Could you check a few things on this model? Use its own coordinates, in mm. Face numbers are marked on the shaded views. Coordinates: 2 decimals unless noted, no trailing zeros. Write each loop counter-clockwise with the first axis right and the second up, starting at its lowest first coordinate (ties: lowest second). Pieces come first, ordered by that corner, then holes.
Item 1: If I drill on probe 1 along Y at (x, z) = (0, 17.25); probe 2 along Y at (x, z) = (0, 20); probe 3 along Y at (x, z) = (-12.25, 18.2), over which ranges is the centre line in solid material (lowest first)?
Item 2: I want a section at A-A on y = 82.8. Please give me the cut outline in (x, z), then the cut area to 3 significant figures.
Item 3: I want a section at B-B on y = -0.2. Please give me the cut outline in (x, z).
Item 4: Thinking about a two-plate mould opening in X: for the marked faces 1, 2, 3 and 4, which applies, +X half, -X half, draft (parallel to the pull), parting line (faces both ways), or undercut?
Item 5: For P1, Ø1.5, axis at y = 64.5, z = 18, coming from the -X side; P2, Ø2.5, axis at x = 0, z = 18.2, coming from the +Y side, each with a flat end and sliding along its axis, tell me the tip position at first contact or that it passes through.
Item 6: I want a section at D-D on z = 18.2. State how many separate pieces and enclosed holes the cut face has, then the cut area to 3 significant figures.
Item 7: I want a section at C-C on x = 0. Please give me the cut outline in (y, z), then the cut area to 3 significant figures.
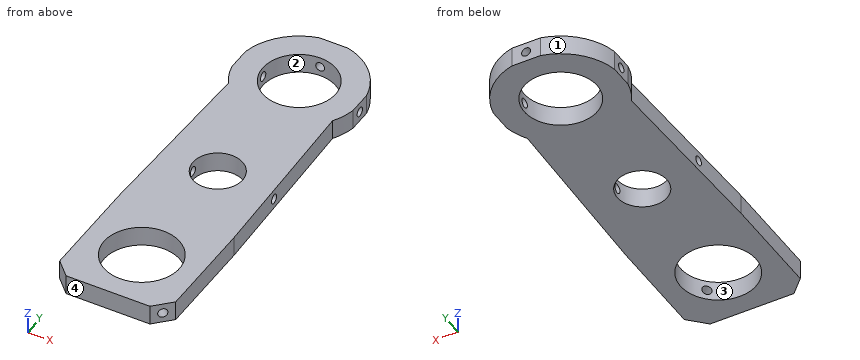
from build123d import *

# Parameters (mm, degrees)
SKETCH002_R          = 7.5
SKETCH002_R_2        = 11.4
SKETCH002_R_3        = 11
PAD002_DEPTH         = 6
SKETCH003_R          = 1.4
POCKET_DEPTH         = 20
SKETCH004_R          = 1.4
POCKET001_DEPTH      = 36.866111375
SKETCH005_R          = 1.4
POCKET002_DEPTH      = 36.6206712513
SKETCH006_R          = 1.35
POCKET003_DEPTH      = 10
BODY_PLACEMENT_ANGLE = 180


with BuildPart() as part:
    # Sketch002 → Pad002 (new body)
    with BuildSketch(Plane.XY):
        with BuildLine():
            Line((17.4185858621, -21.7716146623), (15.72, 32.8960215672))
            ThreePointArc((15.72, 32.8960215672), (17.3549083149, 36.0552761319), (18.3596204304, 39.4676606599))
            Line((18.3596204304, 39.4676606599), (18.3596204304, 46.5323393401))
            ThreePointArc((18.3596204304, 46.5323393401), (13.5034413002, 55.9064608862), (4.3329172916, 61.1369598984))
            Line((-4.3329172916, 61.1369598984), (4.3329172916, 61.1369598984))
            ThreePointArc((-4.3329172916, 61.1369598984), (-13.4407809455, 55.8794757058), (-18.2600508209, 46.5323393401))
            Line((-18.2600508209, 39.4676606599), (-18.2600508209, 46.5323393401))
            ThreePointArc((-18.2600508209, 39.4676606599), (-17.2898053647, 36.137342842), (-15.72, 33.0441076213))
            Line((-17.4185858621, -21.7716146623), (-15.72, 33.0441076213))
            Line((-17.4185858621, -52.4548343373), (-17.4185858621, -21.7716146623))
            Line((-17.4185858621, -52.4548343373), (-12.4548343373, -57.4185858621))
            Line((-12.4548343373, -57.4185858621), (12.8963534851, -57.4185858621))
            Line((17.4185858621, -52.8963534851), (12.8963534851, -57.4185858621))
            Line((17.4185858621, -52.8963534851), (17.4185858621, -21.7716146623))
        make_face()
        Circle(SKETCH002_R, mode=Mode.SUBTRACT)
        with Locations((0, -40)):
            Circle(SKETCH002_R_2, mode=Mode.SUBTRACT)
        with Locations((0.0652183529, 43)):
            Circle(SKETCH002_R_3, mode=Mode.SUBTRACT)
    extrude(amount=PAD002_DEPTH)

    # Sketch003 (on Face12 of Pad002) → Pocket (cut)
    with BuildSketch(Plane(origin=(-34.9367100997, -34.9367100997, 0), x_dir=(0.7071067812, -0.7071067812, 0), z_dir=(-0.7071067812, -0.7071067812, 0))):
        with Locations((28.2842712475, 3)):
            Circle(SKETCH003_R)
    extrude(amount=-POCKET_DEPTH, mode=Mode.SUBTRACT)

    # Sketch004 (on Face14 of Pocket) → Pocket001 (cut, through all)
    with BuildSketch(Plane(origin=(-16.7278822151, 0.5183502661, 0), x_dir=(-0.0309723357, -0.9995202421, 0), z_dir=(-0.9995202421, 0.0309723357, 0))):
        with Locations((0, 3)):
            Circle(SKETCH004_R)
    extrude(amount=-POCKET001_DEPTH, mode=Mode.SUBTRACT)

    # Sketch005 (on Face13 of Pocket001) → Pocket002 (cut, through all)
    with BuildSketch(Plane(origin=(-18.2600508209, 0, 0), x_dir=(0, -1, 0), z_dir=(-1, 0, 0))):
        with Locations((-43, 3)):
            Circle(SKETCH005_R)
    extrude(amount=-POCKET002_DEPTH, mode=Mode.SUBTRACT)

    # Sketch006 (on Face11 of Pocket002) → Pocket003 (cut)
    with BuildSketch(Plane(origin=(0, 61.1369598984, 0), x_dir=(-1, 0, 0), z_dir=(0, 1, 0))):
        with Locations((0, 3)):
            Circle(SKETCH006_R)
    extrude(amount=-POCKET003_DEPTH, mode=Mode.SUBTRACT)


with BuildPart() as part_1:
    # Body002 placement: moved
    add(part.part.moved(Location((0, 39.8, -51))))


with BuildPart() as part_2:
    # Body placement: moved
    add(part_1.part.moved(Location((0, 0, -29.8))).rotate(Axis((0, 0, -29.8), (0, 1, 0)), BODY_PLACEMENT_ANGLE))


solid = part_2.part
Response values:
1. probe 1: y = -17.62 to -11.6, 11.2 to 32.3, 47.3 to 71.8
1. probe 2: y = -17.62 to -11.6, 11.2 to 32.3, 47.3 to 71.8, 93.8 to 100.94
1. probe 3: y = -17.62 to 38.02, 40.82 to 81.4, 84.2 to 96.9
2. outline: (-18.36, 15.2) - (-11.07, 15.2) - (-11.07, 16.8) - (-18.36, 16.8) - close; (-18.36, 19.6) - (-11.07, 19.6) - (-11.07, 21.2) - (-18.36, 21.2) - close; (10.93, 15.2) - (18.26, 15.2) - (18.26, 16.8) - (10.93, 16.8) - close; (10.93, 19.6) - (18.26, 19.6) - (18.26, 21.2) - (10.93, 21.2) - close
2. area: 46.8 mm2
3. outline: (-17.42, 15.2) - (-11.4, 15.2) - (-11.4, 21.2) - (-17.42, 21.2) - close; (11.4, 15.2) - (17.42, 15.2) - (17.42, 21.2) - (11.4, 21.2) - close
4. face 1: -X half
4. face 2: undercut
4. face 3: undercut
4. face 4: draft
5. P1: stops at x = -16
5. P2: stops at y = 71.88
6. separate pieces: 4
6. enclosed holes: 0
6. area: 2,820 mm2
7. outline: (-17.62, 15.2) - (-11.6, 15.2) - (-11.6, 21.2) - (-17.62, 21.2) - close; (11.2, 15.2) - (32.3, 15.2) - (32.3, 21.2) - (11.2, 21.2) - close; (47.3, 15.2) - (71.8, 15.2) - (71.8, 21.2) - (47.3, 21.2) - close; (93.8, 15.2) - (100.94, 15.2) - (100.94, 16.85) - (93.8, 16.85) - close; (93.8, 19.55) - (100.94, 19.55) - (100.94, 21.2) - (93.8, 21.2) - close
7. area: 333 mm2
